from build123d import *

# Parameters (mm, degrees)
SKETCH1_W           = 4.980670257
SKETCH1_H           = 54.9718421
BOSS_EXTRUDE1_DEPTH = 6
SKETCH2_W           = 1.580670257
SKETCH2_H           = 8
CUT_EXTRUDE2_DEPTH  = 7
SKETCH4_W           = 1.580670257
SKETCH4_H           = 25.78592105
CUT_EXTRUDE3_DEPTH  = 7


with BuildPart() as part:
    # Sketch1 → Boss-Extrude1 (new body)
    with BuildSketch(Plane(origin=(0, 0, 0), x_dir=(1, 0, 0), z_dir=(0, 1, 0))):
        with Locations((-11.806033203, 3.043742935)):
            Rectangle(SKETCH1_W, SKETCH1_H)
    extrude(amount=BOSS_EXTRUDE1_DEPTH)

    # Sketch2 → Cut-Extrude2 (cut)
    with BuildSketch(Plane(origin=(0, 6, 0), x_dir=(1, 0, 0), z_dir=(0, 1, 0))):
        with Locations((-11.806033203, 24.829663985)):
            Rectangle(SKETCH2_W, SKETCH2_H)
    extrude(amount=-CUT_EXTRUDE2_DEPTH, mode=Mode.SUBTRACT)

    # Sketch4 → Cut-Extrude3 (cut)
    with BuildSketch(Plane.XZ):
        with Locations((-11.806033203, 9.84921759)):
            Rectangle(SKETCH4_W, SKETCH4_H)
    extrude(amount=-CUT_EXTRUDE3_DEPTH, mode=Mode.SUBTRACT)


solid = part.part
For this review, take the finished solid that the model builds, in its own axes (mm). A direction names the side the tool comes from. Give positions to 0.01 mm unless a question says otherwise; leave off trailing zeros. Order: outer loops, then holes, each group sorted by start corner. A loop starts at its lowest first (then second) coordinate and runs counter-clockwise, first axis right, second up. Notation, with made-up numbers: M -35,-10 L 20,-10 A22 ccw 20,26 Z; hole C -32.5,36.5 d7. An arc over 180 degrees is marked long. Answer in a Markdown table with one row per item. Add a question column.
(1) Consider section A-A on z = 8. State the section outline as (x, y) points, and give its area (3 significant figures).
(2) Wall thickness on probe 1 along Z at (x, y) = (-12, 2.6); probe 2 along X at (y, z) = (1.7, 10): over which ranges is each line inside the solid? List them lowest first. Write a range as [from, to].
(3) Mouldability with a two-part tool opening along Z and no side actions: class faces 1 (the face through (-12, 3, -3.044)), 2 (the face through (-12, 3, -30.53)), 3 (the face through (-12, 3, 24.442)) as +Z half, -Z half, draft (parallel to the pull), parting line (faces both ways), or undercut.
(4) Consider section B-B on x = -11.95. State the section outline as (y, z) points.
(5) For faces 4 (the face through (-9.316, 3, -3)), 5 (the face through (-11.016, 3, -25)), list the 3-axis set-ups (+Z, -Z, +X, -X, +Y, -Y) from which the entire face can be reached by the end or side of a thin tool; tool diameter is ignored.
(6) Consider section C-C on y = 5.15. State the section outline as (x, z) points, and give its area (3 significant figures).
Evaluation:
| question | item | result |
|---|---|---|
| 1 | outline | M -14.3,0 L -12.6,0 L -12.6,6 L -14.3,6 Z; M -11.02,0 L -9.32,0 L -9.32,6 L -11.02,6 Z |
| 1 | area | 20.4 mm^2 |
| 2 | probe 1 | z = [-30.53, -28.83], [-20.83, -3.04], [22.74, 24.44] |
| 2 | probe 2 | x = [-14.3, -12.6], [-11.02, -9.32] |
| 3 | face 1 | undercut |
| 3 | face 2 | -Z half |
| 3 | face 3 | +Z half |
| 4 | outline | M 0,-30.53 L 6,-30.53 L 6,-28.83 L 0,-28.83 Z; M 0,-20.83 L 6,-20.83 L 6,-3.04 L 0,-3.04 Z; M 0,22.74 L 6,22.74 L 6,24.44 L 0,24.44 Z |
| 5 | face 4 | +Z, -Z, +X, +Y, -Y |
| 5 | face 5 | +Y, -Y |
| 6 | outline | M -14.3,-30.53 L -9.32,-30.53 L -9.32,24.44 L -14.3,24.44 Z; hole M -12.6,-28.83 L -11.02,-28.83 L -11.02,-20.83 L -12.6,-20.83 Z; hole M -12.6,-3.04 L -11.02,-3.04 L -11.02,22.74 L -12.6,22.74 Z |
| 6 | area | 220 mm^2 |
